Could you check a few things on this model? Use its own coordinates, in mm. Face numbers are marked on the shaded views. Coordinates: 2 decimals unless noted, no trailing zeros. Loops run counter-clockwise (first coordinate to the right, second up) from the corner with the lowest first, then second, coordinate; pieces in that order, holes last. Notation, with made-up numbers: (26.5, 46) -> (74.5, 46) arc R12 cw to (74.5, 61) -> close; hole circle Ø5 at (27, 59.25). An arc over 180 degrees is marked (long way). One line per question, with ' | ' between items.
from build123d import *

# Parameters (mm, degrees)
SKETCH_1_R               = 55
SKETCH_1_R_2             = 45.5
EXTRUDE_1_DEPTH          = 9
SKETCH_2_R               = 1.75
CUT_EXTRUDE_1_DEPTH      = 9
PATTERN_CIRCULAR_1_COUNT = 6


with BuildPart() as part:
    # 草图1 → 凸台-拉伸1 (new body)
    with BuildSketch(Plane.XY):
        Circle(SKETCH_1_R)
        Circle(SKETCH_1_R_2, mode=Mode.SUBTRACT)
    extrude(amount=EXTRUDE_1_DEPTH)

    # 草图2 → 切除-拉伸1 (cut)
    with BuildSketch(Plane.XY.offset(9)):
        with Locations((0, 52.5)):
            Circle(SKETCH_2_R)
    cut_extrude_1 = extrude(amount=-CUT_EXTRUDE_1_DEPTH, mode=Mode.SUBTRACT)

    # 阵列(圆周)1: 切除-拉伸1 ×6 about axis
    pattern_circular_1_axis = Axis((0, 0, 0), (0, 0, 1))
    for i in range(1, PATTERN_CIRCULAR_1_COUNT):
        add(cut_extrude_1.rotate(pattern_circular_1_axis, i * 360 / PATTERN_CIRCULAR_1_COUNT), mode=Mode.SUBTRACT)

    # 草图3 → 切除-旋转1 (revolve, cut)
    with BuildSketch(Plane(origin=(0, 0, 0), x_dir=(1, 0, 0), z_dir=(0, 1, 0))):
        Polygon((-49.8, 0), (-49.8, -5), (-46.83072822, -5), (-45.5, -5), (-45.5, 0), align=None)
    revolve(axis=Axis((0, 0, 0), (0, 0, 1)), mode=Mode.SUBTRACT)


solid = part.part
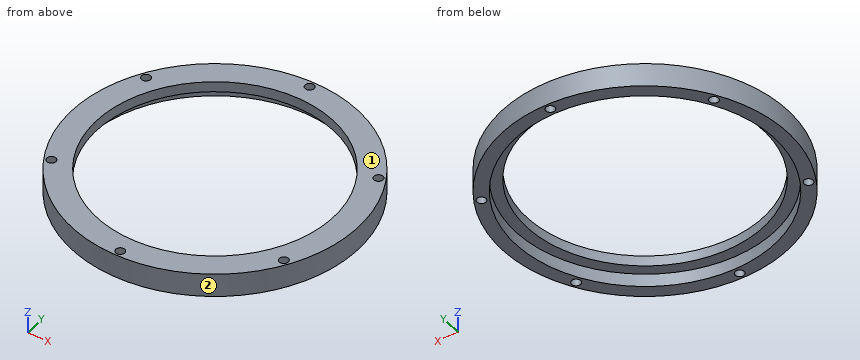
1) We'd pull the mould along X, two halves only. Please class the marked faces 1 and 2: pulls with the +X half, pulls with the -X half, needs draft (parallel to the pull), parting line crosses it, or undercut.
Data:
face 1: needs draft | face 2: parting line crosses it
2) I'm going to push flat-ended pins straight in: pin 1 Ø3 at (y, z) = (-9.5, 5.5) entering from +X; pin 2 Ø2 at (y, z) = (-2.5, 7) entering from +X; pin 3 Ø4.5 at (x, y) = (-45.47, -26.25) entering from +Z; pin 4 Ø3 at (x, y) = (45.47, 26.25) entering from -Z. Where does each tip first touch, or does it pass through?
Data:
pin 1: x = 54.42 | pin 2: x = 54.98 | pin 3: z = 9 | pin 4: through
3) If we section it at D-D on z = 1.25: Please give me the cut outline in (x, y), and give its area (3 significant figures).
Data:
outline: circle Ø110 at (0, 0); hole circle Ø99.6 at (0, 0); hole circle Ø3.5 at (-45.47, -26.25); hole circle Ø3.5 at (-45.47, 26.25); hole circle Ø3.5 at (0, -52.5); hole circle Ø3.5 at (0, 52.5); hole circle Ø3.5 at (45.47, -26.25); hole circle Ø3.5 at (45.47, 26.25) | area: 1,650 mm²
4) I need wall thicknesses on line 1 along Y through (x, z) = (0, 3.6); line 2 along Y through (x, z) = (0, 7.75); line 3 along X through (y, z) = (-26, 5.25). Which ranges of each line are inside material? Lowest first, please. Write a range as from..to.
Data:
line 1: -55..-54.25, -50.75..-49.8, 49.8..50.75, 54.25..55 | line 2: -55..-54.25, -50.75..-45.5, 45.5..50.75, 54.25..55 | line 3: -48.47..-47.2, -43.73..-37.34, 37.34..43.73, 47.2..48.47
5) If we section it at C-C on x = 22.5: Please give me the cut outline in (y, z), and give its area (3 significant figures).
Data:
outline: (-50.19, 0) -> (-44.43, 0) -> (-44.43, 5) -> (-39.55, 5) -> (-39.55, 9) -> (-50.19, 9) -> close; (39.55, 5) -> (44.43, 5) -> (44.43, 0) -> (50.19, 0) -> (50.19, 9) -> (39.55, 9) -> close | area: 143 mm²
6) If we section it at B-B on x = 0: Please give me the cut outline in (y, z).
Data:
outline: (-55, 0) -> (-54.25, 0) -> (-54.25, 9) -> (-55, 9) -> close; (-50.75, 0) -> (-49.8, 0) -> (-49.8, 5) -> (-45.5, 5) -> (-45.5, 9) -> (-50.75, 9) -> close; (45.5, 5) -> (49.8, 5) -> (49.8, 0) -> (50.75, 0) -> (50.75, 9) -> (45.5, 9) -> close; (54.25, 0) -> (55, 0) -> (55, 9) -> (54.25, 9) -> close
7) If we section it at A-A on y = 0: Please give me the cut outline in (x, z).
Data:
outline: (-55, 0) -> (-49.8, 0) -> (-49.8, 5) -> (-45.5, 5) -> (-45.5, 9) -> (-55, 9) -> close; (45.5, 5) -> (49.8, 5) -> (49.8, 0) -> (55, 0) -> (55, 9) -> (45.5, 9) -> close
